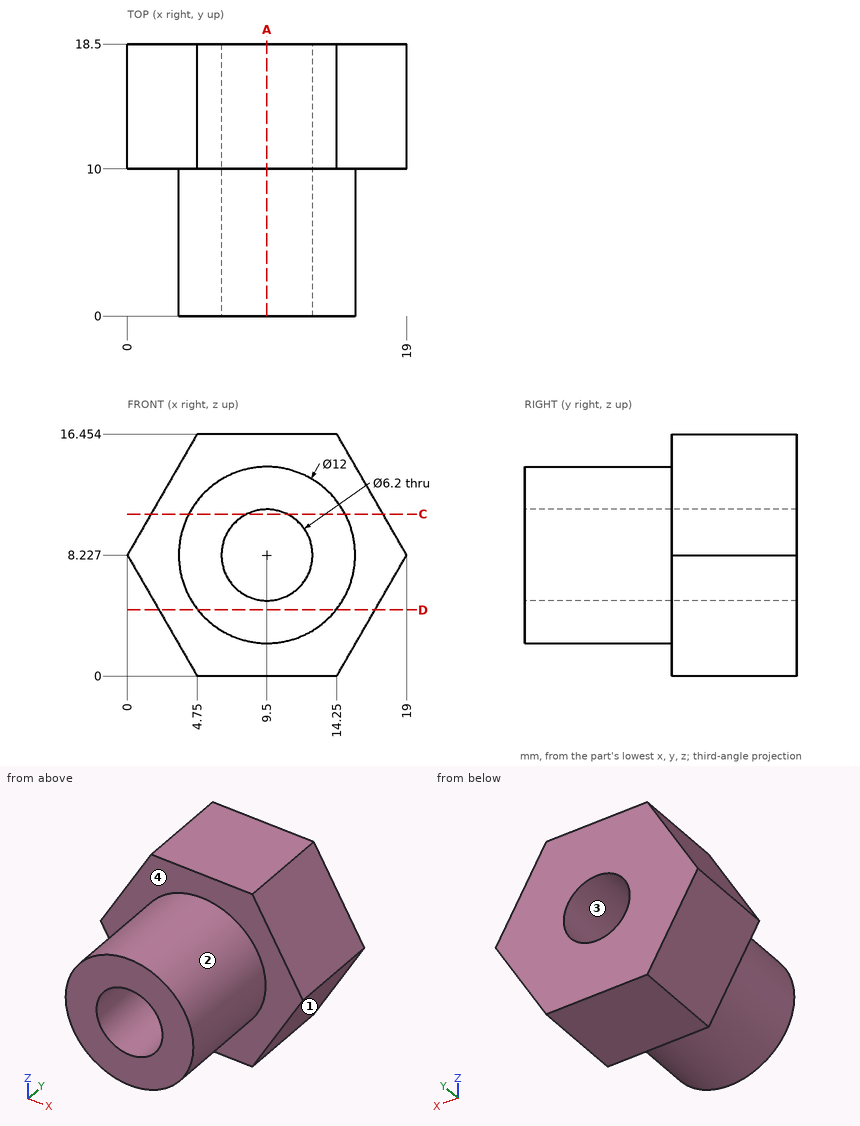
Answer from the drawing. Dimensions are ordinates in mm from the lowest x, y and z of the part. Coordinates: 2 decimals unless noted, no trailing zeros. Loops run counter-clockwise (first coordinate to the right, second up) from the corner with the lowest first, then second, coordinate; pieces in that order, holes last.
Q1. The mould has two halves that part along X. Classify the marked faces 1, 2, 3 and 4: +X half, -X half, draft (parallel to the pull), parting line (faces both ways), or undercut.
Q2. Each of these flat-tipped pins is pushed along its axis until it touches: pin 1 Ø6 at (x, y) = (11, 5) entering from +Z; pin 2 Ø4 at (x, y) = (8.5, 9) entering from -Z; pin 3 Ø8 at (y, z) = (14, 2.5) entering from -X; pin 4 Ø10 at (x, y) = (3, 2) entering from -Z. Where does it stop, or does it pass through?
Q3. The part is cut by section C-C on z = 11. Write down the section's boundary in (x, y).
Q4. The part is cut by section A-A on x = 9.5. Write down the section's boundary in (y, z) (1 decimal), and give its area (3 significant figures).
Q5. Consider probe 1 along Z at (x, y) = (9.5, 7.75); probe 2 along Z at (x, y) = (9.5, 14.25) (1 decimal); probe 3 along X at (y, z) = (4.5, 8.25). Determine where each line is inside the solid, lowest interval first.
Q6. The part is cut by section D-D on z = 4.5. Write down the section's boundary in (x, y), and give its area (3 significant figures).
Results below:
1. face 1: +X half
1. face 2: parting line
1. face 3: undercut
1. face 4: draft
2. pin 1: stops at z = 14.23
2. pin 2: stops at z = 0
2. pin 3: stops at x = 1
2. pin 4: stops at z = 2.42
3. outline: (1.6, 10) - (4.18, 10) - (4.18, 0) - (8.11, 0) - (8.11, 18.5) - (1.6, 18.5) - close; (10.89, 0) - (14.82, 0) - (14.82, 10) - (17.4, 10) - (17.4, 18.5) - (10.89, 18.5) - close
4. outline: (0, 2.2) - (10, 2.2) - (10, 0) - (18.5, 0) - (18.5, 5.1) - (0, 5.1) - close; (0, 11.3) - (18.5, 11.3) - (18.5, 16.5) - (10, 16.5) - (10, 14.2) - (0, 14.2) - close
4. area: 145 mm2
5. probe 1: z = 2.23 to 5.13, 11.33 to 14.23
5. probe 2: z = 0 to 5.1, 11.3 to 16.5
5. probe 3: x = 3.5 to 6.4, 12.6 to 15.5
6. outline: (2.15, 10) - (4.8, 10) - (4.8, 0) - (14.2, 0) - (14.2, 10) - (16.85, 10) - (16.85, 18.5) - (2.15, 18.5) - close
6. area: 219 mm2
